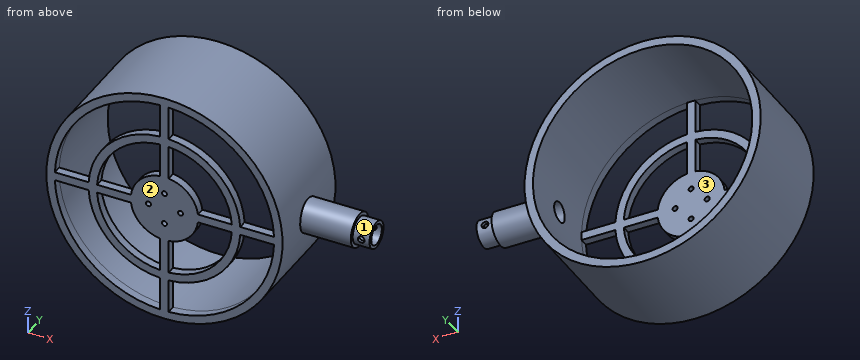
from build123d import *

# Parameters (mm, degrees)
SKETCH1_R                = 70
SKETCH1_R_2              = 65
BOSS_EXTRUDE2_DEPTH      = 60
SKETCH3_R                = 65
BOSS_EXTRUDE4_DEPTH      = 5
CUT_EXTRUDE1_START       = -5
CUT_EXTRUDE1_DEPTH       = 5
SKETCH5_R                = 1.5
CUT_EXTRUDE2_DEPTH       = 5
SKETCH6_R                = 45
SKETCH6_R_2              = 40
BOSS_EXTRUDE5_DEPTH      = 5
BOSS_EXTRUDE7_DEPTH      = 30
BOSS_EXTRUDE7_DEPTH_BACK = 5
SKETCH8_R                = 10
SKETCH10_R               = 7.9
BOSS_EXTRUDE8_DEPTH      = 10
SKETCH11_R               = 6
CUT_EXTRUDE4_DEPTH       = 50
SKETCH13_R               = 2
CUT_EXTRUDE5_DEPTH       = 50


with BuildPart() as part:
    # Sketch1 → Boss-Extrude2 (new body)
    with BuildSketch(Plane(origin=(0, 0, 0), x_dir=(1, 0, 0), z_dir=(0, 1, 0))):
        with Locations(Location((0, 0, 0), (0, 0, 270))):
            Circle(SKETCH1_R)
        with Locations(Location((0, 0, 0), (0, 0, 270))):
            Circle(SKETCH1_R_2, mode=Mode.SUBTRACT)
    extrude(amount=BOSS_EXTRUDE2_DEPTH)

    # Sketch3 → Boss-Extrude4 (add)
    with BuildSketch(Plane(origin=(0, 0, 0), x_dir=(-1, 0, 0), z_dir=(0, -1, 0))):
        with Locations(Location((0, 0, 0), (0, 0, 90))):
            Circle(SKETCH3_R)
    extrude(amount=-BOSS_EXTRUDE4_DEPTH)

    # Sketch4 → Cut-Extrude1 (cut)
    with BuildSketch(Plane(origin=(0, 5, 0), x_dir=(1, 0, 0), z_dir=(0, 1, 0)).offset(CUT_EXTRUDE1_START)):
        with BuildLine():
            ThreePointArc((2.5, 19.843134833), (14.142135624, 14.142135624), (19.843134833, 2.5))
            Line((19.843134833, 2.5), (64.951905284, 2.5))
            ThreePointArc((64.951905284, 2.5), (45.961940777, 45.961940777), (2.5, 64.951905284))
            Line((2.5, 64.951905284), (2.5, 19.843134833))
        make_face()
        with BuildLine():
            ThreePointArc((-19.843134833, 2.5), (-14.141970876, 14.14230037), (-2.499537679, 19.843193074))
            Line((-2.499537679, 19.843193074), (-2.499537679, 64.951923077))
            ThreePointArc((-2.499537679, 64.951923077), (-45.961777201, 45.962104353), (-64.951905284, 2.5))
            Line((-64.951905284, 2.5), (-19.843134833, 2.5))
        make_face()
        with BuildLine():
            Line((64.951905284, -2.5), (19.843134833, -2.5))
            ThreePointArc((19.843134833, -2.5), (14.142135624, -14.142135624), (2.5, -19.843134833))
            Line((2.5, -19.843134833), (2.5, -64.951905284))
            ThreePointArc((2.5, -64.951905284), (45.961940777, -45.961940777), (64.951905284, -2.5))
        make_face()
        with BuildLine():
            Line((-2.499537679, -64.951923077), (-2.499537679, -19.843193074))
            ThreePointArc((-2.499537679, -19.843193074), (-14.141970876, -14.14230037), (-19.843134833, -2.5))
            Line((-19.843134833, -2.5), (-64.951905284, -2.5))
            ThreePointArc((-64.951905284, -2.5), (-45.961777201, -45.962104353), (-2.499537679, -64.951923077))
        make_face()
    extrude(amount=CUT_EXTRUDE1_DEPTH, mode=Mode.SUBTRACT)

    # Sketch5 → Cut-Extrude2 (cut)
    with BuildSketch(Plane(origin=(0, 5, 0), x_dir=(1, 0, 0), z_dir=(0, 1, 0))):
        with Locations(Location((0, 9.5, 0), (0, 0, 270))):
            Circle(SKETCH5_R)
        with Locations(Location((9.5, 0, 0), (0, 0, 270))):
            Circle(SKETCH5_R)
        with Locations(Location((0, -9.5, 0), (0, 0, 270))):
            Circle(SKETCH5_R)
        with Locations(Location((-9.5, 0, 0), (0, 0, 270))):
            Circle(SKETCH5_R)
    extrude(amount=-CUT_EXTRUDE2_DEPTH, mode=Mode.SUBTRACT)

    # Sketch6 → Boss-Extrude5 (add)
    with BuildSketch(Plane(origin=(0, 5, 0), x_dir=(1, 0, 0), z_dir=(0, 1, 0))):
        Circle(SKETCH6_R)
        Circle(SKETCH6_R_2, mode=Mode.SUBTRACT)
    extrude(amount=-BOSS_EXTRUDE5_DEPTH)

    # Sketch8 → Boss-Extrude7 (add, two sides: drawn at the far end of the back side and taken through both)
    with BuildSketch(Plane(origin=(70, 0, 0), x_dir=(0, 0, -1), z_dir=(1, 0, 0)).offset(-BOSS_EXTRUDE7_DEPTH_BACK)):
        with Locations(Location((0, 30, 0), (0, 0, 180))):
            Circle(SKETCH8_R)
    extrude(amount=BOSS_EXTRUDE7_DEPTH + BOSS_EXTRUDE7_DEPTH_BACK)

    # Sketch10 → Boss-Extrude8 (add)
    with BuildSketch(Plane(origin=(100, 0, 0), x_dir=(0, 0, -1), z_dir=(1, 0, 0))):
        with Locations((0, 30)):
            Circle(SKETCH10_R)
    extrude(amount=BOSS_EXTRUDE8_DEPTH)

    # Sketch11 → Cut-Extrude4 (cut)
    with BuildSketch(Plane(origin=(110, 0, 0), x_dir=(0, 0, -1), z_dir=(1, 0, 0))):
        with Locations((0, 30)):
            Circle(SKETCH11_R)
    extrude(amount=-CUT_EXTRUDE4_DEPTH, mode=Mode.SUBTRACT)

    # Sketch13 → Cut-Extrude5 (cut)
    with BuildSketch(Plane(origin=(110, 37.9, 0), x_dir=(1, 0, 0), z_dir=(0, 1, 0))):
        with Locations(Location((-5, 0, 0), (0, 0, 270))):
            Circle(SKETCH13_R)
    extrude(amount=-CUT_EXTRUDE5_DEPTH, mode=Mode.SUBTRACT)


solid = part.part
The model under review builds one solid part; all positions refer to its coordinate system, in mm. Face numbers are marked on the shaded views. Round coordinates to 2 decimals unless told otherwise and drop trailing zeros. Loops run counter-clockwise (first coordinate to the right, second up) from the corner with the lowest first, then second, coordinate; pieces in that order, holes last. Notation, with made-up numbers: M 3.25,-3 L 16.25,-3 A4 cw 16.25,3 Z; hole C -37,9.5 d3. An arc over 180 degrees is marked long. Answer as a JSON object with one key per item and string values.
Item 1: We need section D-D, the plane x = 97. State the section outline as (y, z) points, and give its area (3 significant figures).
Check sheet entries:
{"outline": "C 30,0 d20; hole C 30,0 d12", "area": "201 mm2"}
Item 2: Clearance check with flat-ended pins moving along their axes: P1, Ø2.5, axis at x = -9.5, z = 0, coming from the -Y side; P2, Ø2.5, axis at y = 2, z = -27, coming from the -X side; P3, Ø5.5, axis at x = 56.5, y = 3, coming from the +Z side; P4, Ø1.5, axis at x = 33.5, y = 1.5, coming from the +Z side. State where each tip first meets the part, or that it passes through.
Check sheet entries:
{"P1": "through", "P2": "x = -65.09", "P3": "z = 44.84", "P4": "z = 61.87"}
Item 3: We need section A-A, the plane x = -35. State the section outline as (y, z) points, and give its area (3 significant figures).
Check sheet entries:
{"outline": "M 0,-60.62 L 60,-60.62 L 60,-54.77 L 0,-54.77 Z; M 0,-28.28 L 5,-28.28 L 5,-19.36 L 0,-19.36 Z; M 0,-2.5 L 5,-2.5 L 5,2.5 L 0,2.5 Z; M 0,19.36 L 5,19.36 L 5,28.28 L 0,28.28 Z; M 0,54.77 L 60,54.77 L 60,60.62 L 0,60.62 Z", "area": "816 mm2"}
Item 4: The part is to be moulded in two halves that separate along Z. For the marked faces 1, 2 and 3, say which applies: +Z half, -Z half, draft (parallel to the pull), parting line (faces both ways), or undercut.
Check sheet entries:
{"face 1": "parting line", "face 2": "draft", "face 3": "undercut"}
Item 5: We need section C-C, the plane x = -58. State the section outline as (y, z) points, and give its area (3 significant figures).
Check sheet entries:
{"outline": "M 0,-39.19 L 60,-39.19 L 60,-29.34 L 0,-29.34 Z; M 0,-2.5 L 5,-2.5 L 5,2.5 L 0,2.5 Z; M 0,29.34 L 60,29.34 L 60,39.19 L 0,39.19 Z", "area": "1,210 mm2"}
Item 6: We need section B-B, the plane y = 42.5. State the section outline as (x, z) points, and give its area (3 significant figures).
Check sheet entries:
{"outline": "C 0,0 d140; hole C 0,0 d130", "area": "2,120 mm2"}
Item 7: For line 1 along X through (y, z) = (22.9, 0); line 2 along X through (y, z) = (3.3, 0); line 3 along Z through (x, y) = (9, 2), list the stretches that pass through material, from the lowest coordinate up.
Check sheet entries:
{"line 1": "-70 to -65, 65 to 103, 107 to 110", "line 2": "-70 to -11, -8 to 8, 11 to 70", "line 3": "-69.42 to -64.37, -44.09 to -38.97, -17.86 to -1.41, 1.41 to 17.86, 38.97 to 44.09, 64.37 to 69.42"}
